from build123d import *

# Parameters (mm, degrees)
F1_DEPTH = 60
F0_W     = 44.673472
F0_H     = 10
F2_DEPTH = 30
F0_W_2   = 17.869388
F0_H_2   = 8.934694
F3_DEPTH = 40
F0_W_3   = 17.869389
F4_DEPTH = 20


with BuildPart() as f1:
    # F0 (on Top) → F1 (new body)
    with BuildSketch(Plane.XY):
        Polygon((16.726474, 8.934694), (-36.881692, 8.934694), (-36.881692, -44.673472), (-19.012303, -44.673472), (-19.012303, -35.738778), (-27.946998, -35.738778), (-27.946998, -10), (-27.946998, 0), (16.726474, 0), align=None)
    extrude(amount=F1_DEPTH)

    # F0 (on Top) → F2 (join)
    with BuildSketch(Plane.XY):
        with Locations((-5.610262, -5)):
            Rectangle(F0_W, F0_H)
    extrude(amount=F2_DEPTH)

    # F0 (on Top) → F3 (join)
    with BuildSketch(Plane.XY):
        with Locations((-10.077609, -40.206125)):
            Rectangle(F0_W_2, F0_H_2)
    extrude(amount=F3_DEPTH)

    # F0 (on Top) → F4 (join)
    with BuildSketch(Plane.XY):
        with Locations((7.791779, -40.206125)):
            Rectangle(F0_W_3, F0_H_2)
    extrude(amount=F4_DEPTH)


solid = f1.part
Can you work these out from the model? Positions are in its coordinate system, mm. A direction names the side the tool comes from. Round coordinates to 2 decimals unless told otherwise and drop trailing zeros. Loops run counter-clockwise (first coordinate to the right, second up) from the corner with the lowest first, then second, coordinate; pieces in that order, holes last. Notation, with made-up numbers: (83.5, -35.75) - (121.5, -35.75) arc R26 cw to (121.5, -1.75) - close; hole circle Ø10 at (3, 32). An arc over 180 degrees is marked (long way). Write item = value, one per line. Start each with the question number.
(1) If we section it at C-C (y = -8): Please give me the cut outline in (x, z), and give its area (3 significant figures).
(2) For faces 1 (the face through (-6, 0, 45)), 2 (the face through (-10, -40, 40)), 3 (the face through (-11, -35.739, 23)), 4 (the face through (-28.3, -11.5, 60)), which set-ups out of +Z, -Z, +X, -X, +Y, -Y let a thin tool reach every point of the face, with its end or its side?
(3) If we section it at A-A (x = -10.5): Please give me the cut outline in (y, z).
(4) If I drill on probe 1 along Y at (x, z) = (-10.5, 22.5); probe 2 along Y at (x, z) = (-21, 32); probe 3 along X at (y, z) = (-23, 20), over which ranges is the centre line in solid material (lowest first)? Write a range as [from, to].
(5) If we section it at D-D (x = 13.5): Please give me the cut outline in (y, z), and give its area (3 significant figures).
(6) For P1, Ø7, axis at x = -9, y = -40, coming from the +Z side; P2, Ø8, axis at y = -21.5, z = 51.5, coming from the +X side; P3, Ø3, axis at x = -2, y = -3.5, coming from the +Z side, each with a flat end and sliding along its axis, tell me the tip position at first contact or that it passes through.
(7) If we section it at B-B (z = 43): Please give me the cut outline in (x, y).
(8) If we mould it in two halves opening along Y, with no side actions, what happens to faces 5 (the face through (-6, -10, 15)), 6 (the face through (-10, 8.935, 30)), 7 (the face through (-19.012, -40, 50))? For each: released by +Y, released by -Y, zero draft, split by the parting line, or undercut.
Ans:
q1.outline = (-36.88, 0) - (16.73, 0) - (16.73, 30) - (-27.95, 30) - (-27.95, 60) - (-36.88, 60) - close
q1.area = 1,880 mm²
q2.face_1 = +Z, +X
q2.face_2 = +Z, +X, -Y
q2.face_3 = +Z, -Z, +X
q2.face_4 = +Z, +X, -X, +Y, -Y
q3.outline = (-44.67, 0) - (-35.74, 0) - (-35.74, 40) - (-44.67, 40) - close; (-10, 0) - (8.93, 0) - (8.93, 60) - (0, 60) - (0, 30) - (-10, 30) - close
q4.probe_1 = [-44.67, -35.74], [-10, 8.93]
q4.probe_2 = [-44.67, -35.74], [0, 8.93]
q4.probe_3 = [-36.88, -27.95]
q5.outline = (-44.67, 0) - (-35.74, 0) - (-35.74, 20) - (-44.67, 20) - close; (-10, 0) - (8.93, 0) - (8.93, 60) - (0, 60) - (0, 30) - (-10, 30) - close
q5.area = 1,010 mm²
q6.P1 = 40
q6.P2 = -27.95
q6.P3 = 30
q7.outline = (-36.88, -44.67) - (-19.01, -44.67) - (-19.01, -35.74) - (-27.95, -35.74) - (-27.95, 0) - (16.73, 0) - (16.73, 8.93) - (-36.88, 8.93) - close
q8.face_5 = undercut
q8.face_6 = released by +Y
q8.face_7 = zero draft
